Autodesk Inventor part; units mm, degrees
ref_plane "YZ Plane" through (0, 0, 0) normal (1, 0, 0) x (0, 1, 0)
ref_plane "XZ Plane" through (0, 0, 0) normal (0, 1, 0) x (-1, 0, 0)
ref_plane "XY Plane" through (0, 0, 0) normal (0, 0, 1) x (1, 0, 0)
sketch "Sketch1" plane through (0, 0, 0) normal (0, 1, 0) x (-1, 0, 0)
  circle A0 centre (0, 0) radius 127
  dimension "d0" = 254
extrude "Extrusion1" add sketch "Sketch1" along normal blind 4
sketch "Sketch2" plane through (0, 4, 0) normal (0, 1, 0) x (1, 0, 0)
  circle A0 centre (0, 0) radius 152.4
  circle A1 centre (0, 0) radius 127
  circle A2 centre (0, 0) radius 127
  dimension "d3" = 304.8
extrude "Extrusion2" add sketch "Sketch2" along normal blind 8 and the other way blind 4
chamfer "Chamfer1" distance 15 angle 25 1 edges at (-127, 12, 0) measured on face at (-143.6873, 12, -2.6061)
properties part number "Placeholder_plate"
The model under review builds one solid part; all positions refer to its coordinate system, in mm. A direction names the side the tool comes from. Coordinates: 2 decimals unless noted, no trailing zeros. Write each loop counter-clockwise with the first axis right and the second up, starting at its lowest first coordinate (ties: lowest second). Pieces come first, ordered by that corner, then holes.
1) Machinability: for faces 4 (the face through (-125, 12, -68)), 5 (the face through (-27.53, 4.5, -123.98)), which of the approach directions +Z, -Z, +X, -X, +Y, -Y give a long, thin tool a straight path to every point of the face, cutting with its end or side? Answer none if there is none.
2) The part is to be moulded in two halves that separate along X. For faces 1 (the face through (-120.94, 6.08, 92.73)), 2 (the face through (2, 0, 2)), 3 (the face through (2, 4, 2)), say which applies: pulls with the +X half, pulls with the -X half, needs draft (parallel to the pull), parting line crosses it, or undercut.
3) We need section A-A on x = 0. State the section outline as (y, z) points.
4) We need section B-B on z = 0. State the section outline as (x, y) points.
5) We need section C-C on y = 9.75. State the section outline as (x, z) points.
6) Clearance check with flat-ended pins moving along their axes: pin 1 Ø5 at (y, z) = (9, -27) entering from -X; pin 2 Ø3 at (x, y) = (-14, 6) entering from -Z; pin 3 Ø5 at (y, z) = (10.5, 105) entering from +X; pin 4 Ø6 at (x, z) = (97.5, -81.5) entering from -Y. State where each tip first meets the part, or that it passes through.
7) To check wall thickness, follow probe 1 along X at (y, z) = (4.45, 0); probe 2 along Y at (x, z) = (27, -107). State the ranges of each line that lie inside material, in increasing order.
Answer list:
1. face 4: +Z, -Z, +X, -X, +Y
1. face 5: +Y
2. face 1: parting line crosses it
2. face 2: needs draft
2. face 3: undercut
3. outline: (0, -152.4) - (12, -152.4) - (12, -142) - (5.01, -127) - (4, -127) - (4, 127) - (5.01, 127) - (12, 142) - (12, 152.4) - (0, 152.4) - close
4. outline: (-152.4, 0) - (152.4, 0) - (152.4, 12) - (142, 12) - (127, 5.01) - (127, 4) - (-127, 4) - (-127, 5.01) - (-142, 12) - (-152.4, 12) - close
5. outline: circle Ø304.8 at (0, 0); hole circle Ø274.35 at (0, 0)
6. pin 1: stops at x = -150.42
6. pin 2: stops at z = -151.89
6. pin 3: stops at x = 112.78
6. pin 4: stops at y = 0
7. probe 1: x = -152.4 to -127, 127 to 152.4
7. probe 2: y = 0 to 4
